Geometry: see drawing. Coordinates: mm, zero at the bounding-box minimum. Coordinates: 2 decimals unless noted, no trailing zeros. Write each loop counter-clockwise with the first axis right and the second up, starting at its lowest first coordinate (ties: lowest second). Pieces come first, ordered by that corner, then holes.
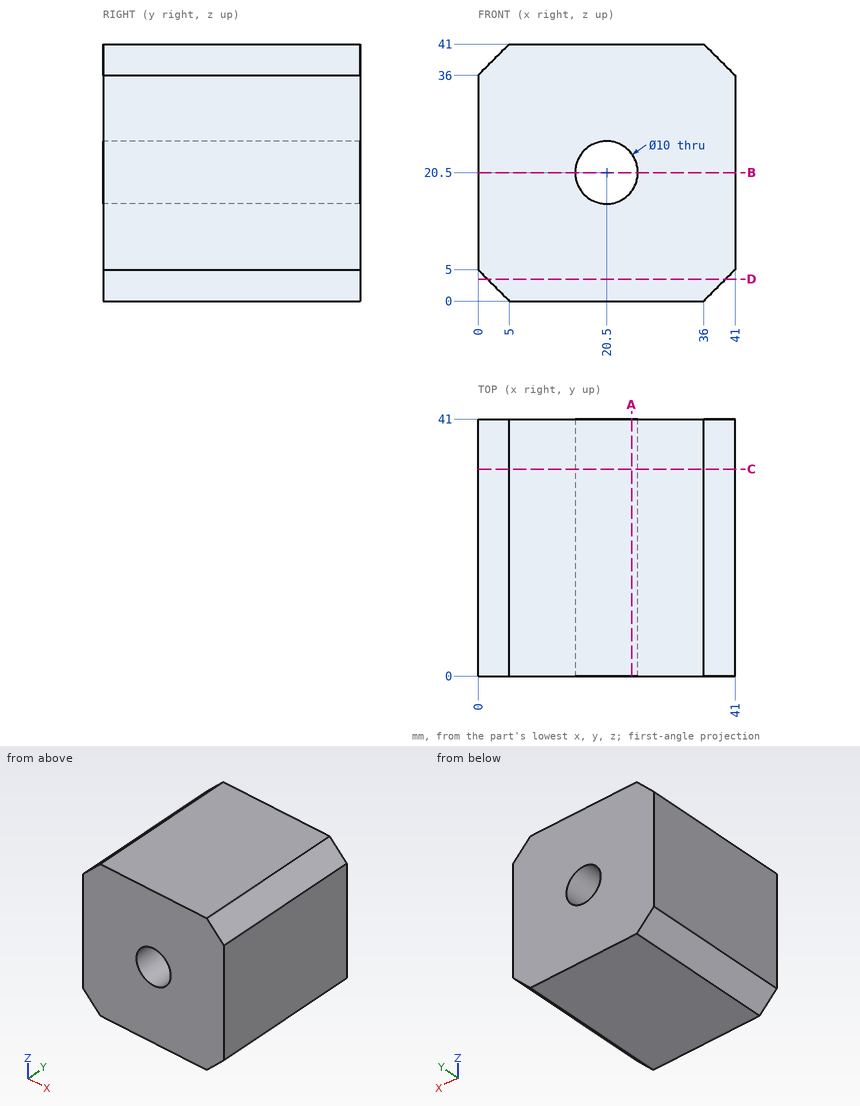
Item 1: Section A-A, the plane x = 24.5. Output: boundary loops of the cut face in (y, z).
Derived:
outline: (0, 0) - (41, 0) - (41, 17.5) - (0, 17.5) - close; (0, 23.5) - (41, 23.5) - (41, 41) - (0, 41) - close
Item 2: Section C-C, the plane y = 33. Output: boundary loops of the cut face in (x, z).
Derived:
outline: (0, 5) - (5, 0) - (36, 0) - (41, 5) - (41, 36) - (36, 41) - (5, 41) - (0, 36) - close; hole circle Ø10 at (20.5, 20.5)
Item 3: Pin query (flat end, axial travel): pin 1 (8 mm diameter, centred on x = 18, z = 35.5, fed in from -Y); pin 2 (5 mm diameter, centred on x = 21.5, z = 21.5, fed in from +Y). Return the tip coordinate at first contact, or that it passes through.
Derived:
pin 1: stops at y = 0
pin 2: passes through
Item 4: Material intervals for probe 1 along X at (y, z) = (21, 23.5); probe 2 along X at (y, z) = (27, 20); probe 3 along Z at (x, y) = (20.5, 17), sorted ascending.
Derived:
probe 1: x = 0 to 16.5, 24.5 to 41
probe 2: x = 0 to 15.53, 25.47 to 41
probe 3: z = 0 to 15.5, 25.5 to 41
Item 5: Section D-D, the plane z = 3.5. Output: boundary loops of the cut face in (x, y).
Derived:
outline: (1.5, 0) - (39.5, 0) - (39.5, 41) - (1.5, 41) - close
Item 6: Section B-B, the plane z = 20.5. Output: boundary loops of the cut face in (x, y).
Derived:
outline: (0, 0) - (15.5, 0) - (15.5, 41) - (0, 41) - close; (25.5, 0) - (41, 0) - (41, 41) - (25.5, 41) - close
